The listing builds one solid part. Answer for the finished solid, in the listing's coordinates (mm). A direction names the side the tool comes from. Coordinates: 2 decimals unless noted, no trailing zeros. Order: outer loops, then holes, each group sorted by start corner. A loop starts at its lowest first (then second) coordinate and runs counter-clockwise, first axis right, second up.
from build123d import *

# Parameters (mm, degrees)
CYLINDER068_R             = 13.9827
CYLINDER068_DEPTH         = 28.0162
CYLINDER067_R             = 13.9827
CYLINDER067_DEPTH         = 32.1945
FUSION026_PLACEMENT_ANGLE = 42.9


with BuildPart() as cylinder068:
    # Cylinder068 → Cylinder068 (new body)
    with BuildSketch(Plane.XZ.offset(-14.0081)):
        Circle(CYLINDER068_R)
    extrude(amount=CYLINDER068_DEPTH)


with BuildPart() as rear_inner_slip_l:
    # Cylinder067 → Cylinder067 (new body)
    with BuildSketch(Plane.XY):
        Circle(CYLINDER067_R)
    extrude(amount=CYLINDER067_DEPTH)

    # Fusion026: union Cylinder068
    add(cylinder068.part)


with BuildPart() as rear_inner_slip_l_1:
    # Fusion026 placement: moved
    add(rear_inner_slip_l.part.moved(Location((-452, -14, -18))).rotate(Axis((-452, -14, -18), (0, 1, 0)), FUSION026_PLACEMENT_ANGLE))


solid = rear_inner_slip_l_1.part
1) Each of these flat-tipped pins is pushed along its axis until it touches: P1, Ø1.5, axis at x = -442.5, z = -5, coming from the +Y side; P2, Ø4, axis at y = -17, z = -9, coming from the -X side; P3, Ø2, axis at x = -445.5, z = -0.5, coming from the -Y side; P4, Ø10, axis at x = -454.5, y = -23.5, coming from the -Z side. Where does it stop, or does it pass through?
2) Consider L1, parallel to Z at x = -429.5, y = -9; L2, parallel to Y at x = -443, z = -4; L3, parallel to X at y = -16.75, z = -22. Determine where each line is inside the solid, lowest interval first.
3) A tool of negligible diameter and unlimited length cuts with its end or side. For faces 1 (the face through (-463.51, -13.8, -25.94)), 2 (the face through (-452, -28.008, -18)), from which of +Z, -Z, +X, -X, +Y, -Y can it reach the whole face along a straight path? Write none if from no direction.
4) Section A-A (y = -20) is taken. Give the vertices of the cut face in (x, z).
5) Section B-B (x = -463) is taken. Give the vertices of the cut face in (y, z).
Filled sheet:
1. P1: stops at y = -0.06
1. P2: stops at x = -464.1
1. P3: stops at y = -26.56
1. P4: stops at z = -31.98
2. L1: z = -12.97 to 5.04
2. L2: y = -27.67 to -0.33
2. L3: x = -465.4 to -437
3. face 1: none
3. face 2: +Z, -Z, +X, -X, -Y
4. outline: (-457.17, -5.01) arc R13.98 ccw (long way) to (-438.66, -22.2) - (-420.83, -3.01) - (-439.34, 14.18) - close
5. outline: (-28.01, -26.63) - (0.01, -26.63) - (0.01, -9.37) - (-28.01, -9.37) - close
